Here's how the part is built. I have some questions about the finished solid (model axes, mm). A direction names the side the tool comes from. Round coordinates to 2 decimals unless told otherwise and drop trailing zeros. Write each loop counter-clockwise with the first axis right and the second up, starting at its lowest first coordinate (ties: lowest second). Pieces come first, ordered by that corner, then holes. Notation, with made-up numbers: (-35, 36.25) -> (5, 36.25) arc R15 ccw to (5, 45.25) -> close; hole circle Ø5 at (-15.75, -9). An arc over 180 degrees is marked (long way). Put each result on its own line as item: value. Start each with the question number.
1) Which directions (+Z, -Z, +X, -X, +Y, -Y) give clear straight access to the entire face, cutting with the end or side of a thin tool? Please do faces 1 (the cylindrical face through (-56.84, 10.89, 107.86)), 2 (the flat face through (-67, 13, 101.6)), 3 (the flat face through (-68, 13, 114.3)), 4 (the flat face through (-66, 25.4, 58)), 5 (the cylindrical face through (-126.911, 14.203, 60.776)).
2) I want a section at D-D, the plane y = 12.7. List the corners of the cut face in (x, z) for me (3 decimals).
3) I want a section at A-A, the plane z = 81.5. List the corners of the cut face in (x, y) for me.
4) I want a section at C-C, the plane x = -29. List the corners of the cut face in (y, z) for me (3 decimals), then the cut area to 3 significant figures.
5) Will this pin go through, and if not, where does the flat tip stop? P1, Ø6.5, axis at x = -60.325, y = 12.7, coming from the +Z side (3 decimals).
6) I want a section at B-B, the plane z = 57.15. List the corners of the cut face in (x, y) for me (3 decimals).
7) We'd pull the mould along X, two halves only. Please class faces 6 (the flat face through (-12.7, 13, 91)), 7 (the flat face through (-133.35, 18, 56)), 8 (the flat face through (-66, 0, 58)), 9 (the flat face through (0, 13, 58)): released by +X, released by -X, zero draft, split by the parting line, or undercut.
8) If I drill on line 1 along X through (y, z) = (22, 15) (3 decimals); line 2 along Z through (x, y) = (-32, 12.5) (3 decimals); line 3 along Z through (x, y) = (-127.5, 12.7) (3 decimals), over which ranges is the centre line in solid material (lowest first)? Write a range as [from, to].
Autodesk Inventor part; units mm, degrees
ref_plane "YZ Plane" through (0, 0, 0) normal (1, 0, 0) x (0, 1, 0)
ref_plane "XZ Plane" through (0, 0, 0) normal (0, 1, 0) x (-1, 0, 0)
ref_plane "XY Plane" through (0, 0, 0) normal (0, 0, 1) x (1, 0, 0)
sketch "Sketch1" plane through (0, 0, 0) normal (0, 1, 0) x (-1, 0, 0)
  line L0 (0, 0) -> (133.35, 0)
  line L1 (133.35, 0) -> (133.35, 114.3)
  line L2 (133.35, 114.3) -> (0, 114.3)
  line L3 (0, 114.3) -> (0, 0)
  line L4 (12.7, 12.7) -> (120.65, 12.7)
  line L5 (120.65, 12.7) -> (120.65, 101.6)
  line L6 (120.65, 101.6) -> (12.7, 101.6)
  line L7 (12.7, 101.6) -> (12.7, 12.7)
  line L8 (12.7, 12.7) -> (98.425, 12.7)
  line L9 (98.425, 12.7) -> (98.425, 79.375)
  line L10 (98.425, 79.375) -> (12.7, 79.375)
  line L11 (12.7, 79.375) -> (12.7, 12.7)
  dimension "d0" = 114.3
  dimension "d1" = 133.35
  dimension "d2" = 12.7
  dimension "d3" = 12.7
  dimension "d4" = 12.7
  dimension "d5" = 12.7
  dimension "d6" = 22.225
  dimension "d7" = 22.225
extrude "Extrusion1" add sketch "Sketch1" along normal blind 25.4 contours L3 L2 L1 L0 | L7 L10 L9 L4
sketch "Sketch3" plane through (-133.35, 0, 114.3) normal (0, 0, 1) x (1, 0, 0)
  line L0 (133.35, 0) -> (133.35, 25.4)
  line L1 (0, 25.4) -> (133.35, 25.4)
  line L2 (12.7, 0) -> (12.7, 25.4)
  point P0 (73.025, 12.7)
  dimension "d10" = 120.65
  dimension "d11" = 25.4
  dimension "d12" = 60.325
  dimension "d13" = 12.7
hole "Hole1" at (-60.325, 12.7, 114.3) direction (0, 0, -1) diameter 7.85 depth 12.7
sketch "Sketch4" plane through (-133.35, 0, 0) normal (-1, 0, 0) x (0, 0, 1)
  line L0 (0, 25.4) -> (114.3, 25.4)
  line L1 (114.3, 0) -> (114.3, 25.4)
  point P0 (0, 0)
  point P1 (57.15, 12.7)
  dimension "d21" = 25.4
  dimension "d22" = 114.3
  dimension "d23" = 12.7
  dimension "d24" = 57.15
hole "Hole2" at (-133.35, 12.7, 57.15) direction (1, 0, 0) diameter 7.85 depth 12.7
equation "\"d3\" = d2"
equation "\"d4\" = d2"
equation "\"d5\" = d2"
equation "\"d6\" = d7"
properties part number "odometery system base"
Findings:
1. face 1: +Z
1. face 2: +Y, -Y
1. face 3: +Z, +X, -X, +Y, -Y
1. face 4: +Z, -Z, +X, -X, +Y
1. face 5: -X
2. outline: (-133.35, 0) -> (0, 0) -> (0, 114.3) -> (-56.4, 114.3) -> (-56.4, 101.6) -> (-12.7, 101.6) -> (-12.7, 79.375) -> (-98.425, 79.375) -> (-98.425, 12.7) -> (-120.65, 12.7) -> (-120.65, 53.225) -> (-133.35, 53.225) -> close; (-133.35, 61.075) -> (-120.65, 61.075) -> (-120.65, 101.6) -> (-64.25, 101.6) -> (-64.25, 114.3) -> (-133.35, 114.3) -> close
3. outline: (-133.35, 0) -> (-120.65, 0) -> (-120.65, 25.4) -> (-133.35, 25.4) -> close; (-12.7, 0) -> (0, 0) -> (0, 25.4) -> (-12.7, 25.4) -> close
4. outline: (0, 0) -> (25.4, 0) -> (25.4, 79.375) -> (0, 79.375) -> close; (0, 101.6) -> (25.4, 101.6) -> (25.4, 114.3) -> (0, 114.3) -> close
4. area: 2,340 mm2
5. P1: stops at z = 79.375
6. outline: (-133.35, 0) -> (-120.65, 0) -> (-120.65, 8.775) -> (-133.35, 8.775) -> close; (-133.35, 16.625) -> (-120.65, 16.625) -> (-120.65, 25.4) -> (-133.35, 25.4) -> close; (-98.425, 0) -> (0, 0) -> (0, 25.4) -> (-98.425, 25.4) -> close
7. face 6: undercut
7. face 7: released by -X
7. face 8: zero draft
7. face 9: released by +X
8. line 1: x = [-133.35, -120.65], [-98.425, 0]
8. line 2: z = [0, 79.375], [101.6, 114.3]
8. line 3: z = [0, 53.225], [61.075, 114.3]
